For this review, use the dimensioned drawing (mm, ordinates from the lowest corner) and the shaded views. Give positions to 0.01 mm unless a question says otherwise; leave off trailing zeros. Write each loop counter-clockwise with the first axis right and the second up, starting at its lowest first coordinate (ties: lowest second). Pieces come first, ordered by that corner, then holes. Notation, with made-up numbers: M 49.5,60 L 64.5,60 A24 ccw 64.5,94 Z; hole C 53,-36 d7. An arc over 180 degrees is marked long. Write each question's results on one line, items separated by ' | '. Start each with the question number.
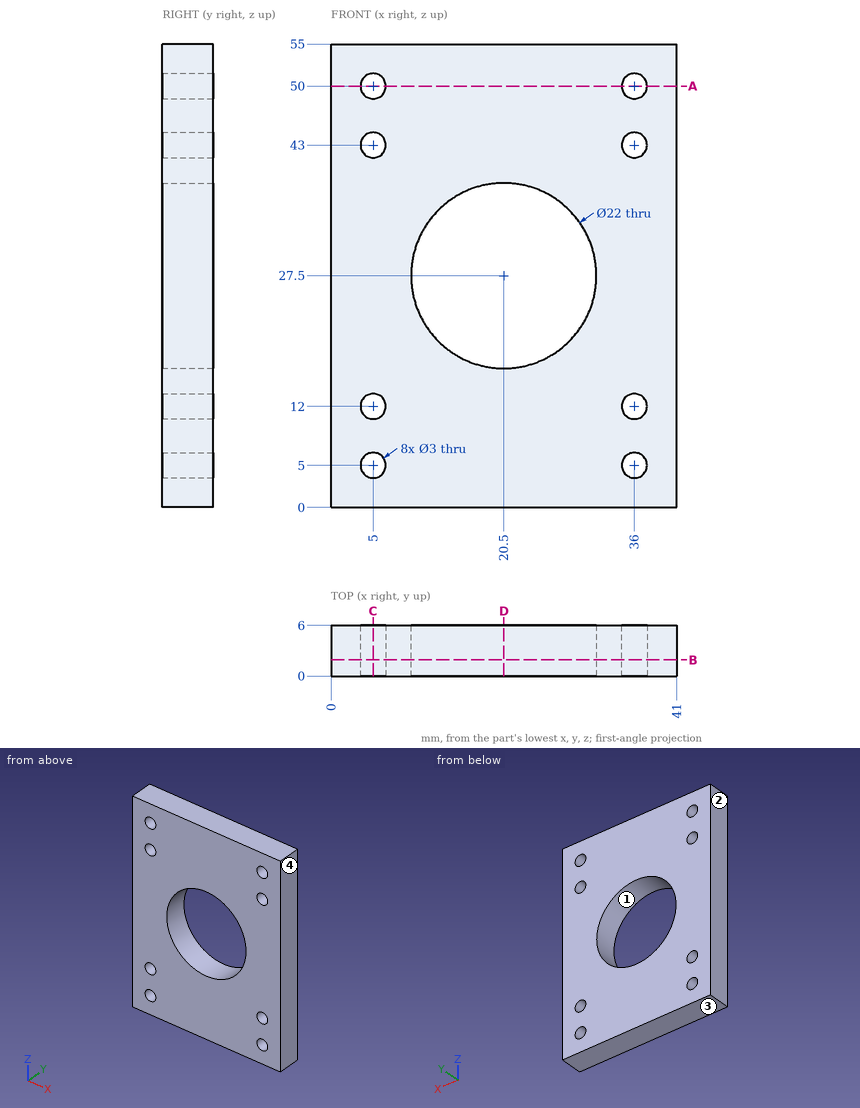
(1) Draft analysis for pull direction X (two halves, no side actions). For the marked faces 1, 2, 3 and 4, state which applies: pulls with the +X half, pulls with the -X half, needs draft (parallel to the pull), parting line crosses it, or undercut.
(2) Add section A-A (z = 50). State the section outline as (x, y) points.
(3) Wall thickness on L1, parallel to Z at x = 36, y = 4; L2, parallel to Z at x = 36.5, y = 2.25; L3, parallel to Z at x = 21.5, y = 3.6: over which ranges is each line inside the solid? List them lowest first.
(4) Add section D-D (x = 20.5). State the section outline as (y, z) points, then the cut area to 3 significant figures.
(5) Add section B-B (y = 1.9). Give the number of separate pieces and of enclosed holes in the cut face, then the cut area to 3 significant figures.
(6) Add section C-C (x = 5). State the section outline as (y, z) points.
(7) Clearance check with a flat-ended pin moving along its axis: P1, Ø1.8, axis at x = 5, z = 5, coming from the +Y side. State where the tip first meets the part, or that it passes through.
Calculated:
1) face 1: undercut | face 2: pulls with the -X half | face 3: needs draft | face 4: pulls with the +X half
2) outline: M 0,0 L 3.5,0 L 3.5,6 L 0,6 Z; M 6.5,0 L 34.5,0 L 34.5,6 L 6.5,6 Z; M 37.5,0 L 41,0 L 41,6 L 37.5,6 Z
3) L1: z = 0 to 3.5, 6.5 to 10.5, 13.5 to 41.5, 44.5 to 48.5, 51.5 to 55 | L2: z = 0 to 3.59, 6.41 to 10.59, 13.41 to 41.59, 44.41 to 48.59, 51.41 to 55 | L3: z = 0 to 16.55, 38.45 to 55
4) outline: M 0,0 L 6,0 L 6,16.5 L 0,16.5 Z; M 0,38.5 L 6,38.5 L 6,55 L 0,55 Z | area: 198 mm²
5) separate pieces: 1 | enclosed holes: 9 | area: 1,820 mm²
6) outline: M 0,0 L 6,0 L 6,3.5 L 0,3.5 Z; M 0,6.5 L 6,6.5 L 6,10.5 L 0,10.5 Z; M 0,13.5 L 6,13.5 L 6,41.5 L 0,41.5 Z; M 0,44.5 L 6,44.5 L 6,48.5 L 0,48.5 Z; M 0,51.5 L 6,51.5 L 6,55 L 0,55 Z
7) P1: passes through
